Input: part model. Units: mm. Frame: model coordinates. A direction names the side the tool comes from. Round coordinates to 2 decimals unless told otherwise and drop trailing zeros. Order: outer loops, then holes, each group sorted by start corner. A loop starts at its lowest first (then second) coordinate and runs counter-clockwise, first axis right, second up.
Item 1: Line query: L1, parallel to Z at x = 0, y = 3.25; L2, parallel to X at y = 4, z = 0; L3, parallel to X at y = 6.25, z = -45. Output: solid intervals per line, ascending.
Item 2: Cut plane D-D on z = 0. Output: boundary loops of the cut face in (x, y).
Item 3: Reachability of faces 4 (the flat face through (12, 5, -39)), 5 (the flat face through (-12, 5, 39)), 6 (the flat face through (12, 5, 39)), 7 (the flat face through (-12, 5, -39)) from +Z, -Z, +X, -X, +Y, -Y: full face, straight path, thin tool, end or side. Return the list, or none.
Item 4: Cut plane C-C on x = 0. Output: boundary loops of the cut face in (y, z), then the cut area to 3 significant figures.
Item 5: Mould query, pull axis X, two halves, no side actions, for faces 1 (the cylindrical face through (0, 5, 57)), 2 (the cylindrical face through (-0.121, 4.93, 25.253)), 3 (the cylindrical face through (18.14, 5.07, -29.1)). Classes: released by +X, released by -X, zero draft, split by the parting line, or undercut.
Item 6: Cut plane B-B on y = 5. Output: boundary loops of the cut face in (x, z), then the cut area to 3 significant figures.
Item 7: Cut plane A-A on z = 28.5. Output: boundary loops of the cut face in (x, y), then the cut area to 3 significant figures.
Item 8: First-contact query: pin 1 (0.5 mm diameter, centred on x = 15.5, y = 6.5, fed in from +Z); pin 2 (11.5 mm diameter, centred on x = 0, z = 0, fed in from -Y); pin 3 (3 mm diameter, centred on y = 5, z = 36.5, fed in from +X); pin 4 (5 mm diameter, centred on y = 6.5, z = -37, fed in from -X). Flat tips, straight axial feed; report the tip coordinate or a pass-through.
Autodesk Inventor part; units mm, degrees
ref_plane "YZ Plane" through (0, 0, 0) normal (1, 0, 0) x (0, 1, 0)
ref_plane "XZ Plane" through (0, 0, 0) normal (0, 1, 0) x (-1, 0, 0)
ref_plane "XY Plane" through (0, 0, 0) normal (0, 0, 1) x (1, 0, 0)
sketch "Sketch1" plane through (0, 0, 0) normal (0, 1, 0) x (-1, 0, 0)
  line L0 (0, 45) -> (0, -45) construction
  line L1 (-12, 45) -> (-12, -45)
  line L2 (12, -45) -> (12, 45)
  arc A0 (12, 45) -> (-12, 45) centre (0, 45) ccw
  arc A1 (-12, -45) -> (12, -45) centre (0, -45) ccw
  line L3 (-19, 30) -> (-19, -30)
  line L4 (-19, -30) -> (19, -30)
  line L5 (19, -30) -> (19, 30)
  line L6 (19, 30) -> (-19, 30)
  line L7 (-19, 30) -> (19, -30) construction
  line L8 (-19, -30) -> (19, 30) construction
  point P0 (0, 0)
  point P1 (-12, 30)
  point P2 (-12, -30)
  point P3 (12, -30)
  point P4 (12, 30)
  dimension "d0" = 60
  dimension "d1" = 90
  dimension "d2" = 12
  dimension "d3" = 38
extrude "Extrusion1" add sketch "Sketch1" along normal blind 10
sketch "Sketch2" plane through (0, 10, 0) normal (0, 1, 0) x (1, 0, 0)
  line L0 (19, -30) -> (19, 30)
  line L1 (19, 30) -> (12, 30)
  line L2 (12, 30) -> (12, 45)
  arc A0 (12, 45) -> (-12, 45) centre (0, 45) ccw
  line L3 (-12, 45) -> (-12, 30)
  line L4 (-12, 30) -> (-19, 30)
  line L5 (-19, 30) -> (-19, -30)
  line L6 (-19, -30) -> (-12, -30)
  line L7 (-12, -30) -> (-12, -45)
  arc A1 (-12, -45) -> (12, -45) centre (0, -45) ccw
  line L8 (12, -45) -> (12, -30)
  line L9 (12, -30) -> (19, -30)
  line L10 (0, -28) -> (0, 28)
  line L11 (0, 0) -> (-19, 0)
  line L12 (-19, 30) -> (-19, -30)
  dimension "d6" = 56
hole "Hole1" at (0, 10, 28) at (0, 10, -28) direction (0, -1, 0) diameter 5.5 end through all
fillet "Fillet1" radius 3 8 edges at (19, 5, 30) (19, 5, -30) (12, 5, 30) (-19, 5, 30) (-12, 5, 30) (-19, 5, -30) (-12, 5, -30) (12, 5, -30)
sketch "Sketch3" plane through (0, 10, 0) normal (0, 1, 0) x (1, 0, 0)
  arc A0 (-12, -45) -> (12, -45) centre (0, -45) ccw
  arc A1 (12, 45) -> (-12, 45) centre (0, 45) ccw
  point P0 (0, 0)
hole "Hole2" at (0, 10, 45) at (0, 10, -45) direction (0, -1, 0) diameter 5.5 end through all
sketch "Sketch4" plane through (0, 10, 0) normal (0, 1, 0) x (1, 0, 0)
  circle A0 centre (0, 0) radius 5
  dimension "d22" = 10
extrude "Extrusion2" cut sketch "Sketch4" against normal blind 7.5
properties part number "11_Mieng_go_dem_lo_xo"
From the geometry:
1. L1: z = -57 to -47.75, -42.25 to -30.75, -25.25 to -5, 5 to 25.25, 30.75 to 42.25, 47.75 to 57
1. L2: x = -19 to -5, 5 to 19
1. L3: x = -12 to -2.75, 2.75 to 12
2. outline: (-19, 0) - (19, 0) - (19, 10) - (5, 10) - (5, 2.5) - (-5, 2.5) - (-5, 10) - (-19, 10) - close
3. face 4: -Z, +X, +Y, -Y
3. face 5: +Z, -X, +Y, -Y
3. face 6: +Z, +X, +Y, -Y
3. face 7: -Z, -X, +Y, -Y
4. outline: (0, -57) - (10, -57) - (10, -47.75) - (0, -47.75) - close; (0, -42.25) - (10, -42.25) - (10, -30.75) - (0, -30.75) - close; (0, -25.25) - (10, -25.25) - (10, -5) - (2.5, -5) - (2.5, 5) - (10, 5) - (10, 25.25) - (0, 25.25) - close; (0, 30.75) - (10, 30.75) - (10, 42.25) - (0, 42.25) - close; (0, 47.75) - (10, 47.75) - (10, 57) - (0, 57) - close
4. area: 845 mm2
5. face 1: split by the parting line
5. face 2: undercut
5. face 3: released by +X
6. outline: (-19, -27) arc R3 ccw to (-16, -30) - (-15, -30) arc R3 cw to (-12, -33) - (-12, -45) arc R12 ccw to (12, -45) - (12, -33) arc R3 cw to (15, -30) - (16, -30) arc R3 ccw to (19, -27) - (19, 27) arc R3 ccw to (16, 30) - (15, 30) arc R3 cw to (12, 33) - (12, 45) arc R12 ccw to (-12, 45) - (-12, 33) arc R3 cw to (-15, 30) - (-16, 30) arc R3 ccw to (-19, 27) - close; hole circle Ø10 at (0, 0); hole circle Ø5.5 at (0, -45); hole circle Ø5.5 at (0, -28); hole circle Ø5.5 at (0, 28); hole circle Ø5.5 at (0, 45)
6. area: 3,280 mm2
7. outline: (-18.6, 0) - (-2.7, 0) - (-2.7, 10) - (-18.6, 10) - close; (2.7, 0) - (18.6, 0) - (18.6, 10) - (2.7, 10) - close
7. area: 318 mm2
8. pin 1: stops at z = 30
8. pin 2: stops at y = 0
8. pin 3: stops at x = 12
8. pin 4: stops at x = -12
